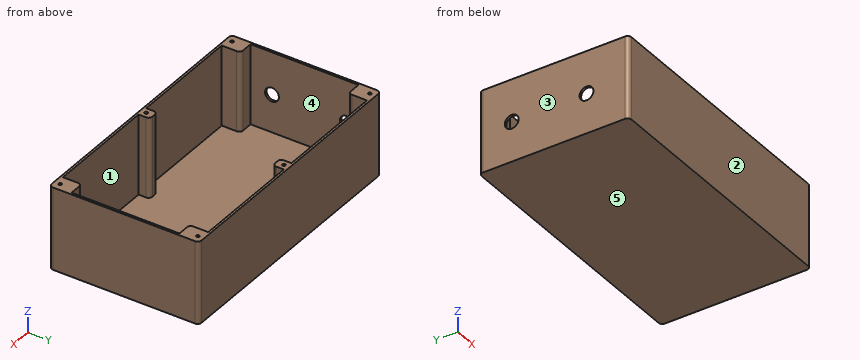
from build123d import *

# Parameters (mm, degrees)
F0_W     = 360
F0_H     = 200
F1_DEPTH = 110
F2_R     = 5
F3_T     = -3
F5_D     = 18.5
F5_DEPTH = 16.5
F5_TIP   = 5.557960726
F8_DEPTH = 107
F9_D     = 4.2
F9_DEPTH = 22.4
F9_TIP   = 1.2618073


with BuildPart() as f1:
    # F0 (on Top) → F1 (new body)
    with BuildSketch(Plane.XY):
        Rectangle(F0_W, F0_H)
    extrude(amount=F1_DEPTH)

    # F2
    f2_edges = [f1.edges().sort_by_distance(p)[0] for p in [
        (-180, 100, 55),
        (-180, -100, 55),
        (180, -100, 55),
        (180, 100, 55),
    ]]
    fillet(f2_edges, radius=F2_R)

    # F3
    f3_openings = [f1.faces().sort_by_distance(p)[0] for p in [
        (0, 0, 110),
    ]]
    offset(amount=F3_T, openings=f3_openings)

    # F5
    with Locations(Plane(origin=(-180, 0, 0), x_dir=(0, -1, 0), z_dir=(-1, 0, 0))):
        with Locations((-56.4456321299, 53.3652417362), (43.4474907815, 53.3652417362)):
            Hole(F5_D / 2, depth=F5_DEPTH)
            with Locations((0, 0, -(F5_DEPTH + F5_TIP / 2))):  # 118° drill point
                Cone(0, F5_D / 2, F5_TIP, mode=Mode.SUBTRACT)

    # F7 (on face) → F8 (join, through all)
    with BuildSketch(Plane.XY.offset(110)):
        with BuildLine():
            Line((-177, 95), (-177, 72))
            Line((-177, 72), (-162, 72))
            ThreePointArc((-162, 72), (-158.4644660941, 73.4644660941), (-157, 77))
            Line((-157, 77), (-157, 97))
            Line((-157, 97), (-175, 97))
            ThreePointArc((-175, 97), (-176.4142135624, 96.4142135624), (-177, 95))
        make_face()
        with BuildLine():
            Line((-175, -97), (-157, -97))
            Line((-157, -97), (-157, -77))
            ThreePointArc((-157, -77), (-158.4644660941, -73.4644660941), (-162, -72))
            Line((-162, -72), (-177, -72))
            Line((-177, -72), (-177, -95))
            ThreePointArc((-177, -95), (-176.4142135624, -96.4142135624), (-175, -97))
        make_face()
        with BuildLine():
            Line((7.5, 87), (7.5, 97))
            Line((7.5, 97), (-7.5, 97))
            Line((-7.5, 97), (-7.5, 87))
            ThreePointArc((-7.5, 87), (-6.0355339059, 83.4644660941), (-2.5, 82))
            Line((-2.5, 82), (2.5, 82))
            ThreePointArc((2.5, 82), (6.0355339059, 83.4644660941), (7.5, 87))
        make_face()
        with BuildLine():
            Line((-7.5, -97), (7.5, -97))
            Line((7.5, -97), (7.5, -87))
            ThreePointArc((7.5, -87), (6.0355339059, -83.4644660941), (2.5, -82))
            Line((2.5, -82), (-2.5, -82))
            ThreePointArc((-2.5, -82), (-6.0355339059, -83.4644660941), (-7.5, -87))
            Line((-7.5, -87), (-7.5, -97))
        make_face()
        with BuildLine():
            Line((157, -97), (175, -97))
            ThreePointArc((175, -97), (176.4142135624, -96.4142135624), (177, -95))
            Line((177, -95), (177, -72))
            Line((177, -72), (162, -72))
            ThreePointArc((162, -72), (158.4644660941, -73.4644660941), (157, -77))
            Line((157, -77), (157, -97))
        make_face()
        with BuildLine():
            Line((162, 72), (177, 72))
            Line((177, 72), (177, 95))
            ThreePointArc((177, 95), (176.4142135624, 96.4142135624), (175, 97))
            Line((175, 97), (157, 97))
            Line((157, 97), (157, 77))
            ThreePointArc((157, 77), (158.4644660941, 73.4644660941), (162, 72))
        make_face()
    extrude(amount=-F8_DEPTH)

    # F9
    with Locations(Plane.XY.offset(110)):
        with Locations((-170, -92), (-170, 92), (0, 92), (170, 92), (170, -92), (0, -92)):
            Hole(F9_D / 2, depth=F9_DEPTH)
            with Locations((0, 0, -(F9_DEPTH + F9_TIP / 2))):  # 118° drill point
                Cone(0, F9_D / 2, F9_TIP, mode=Mode.SUBTRACT)


solid = f1.part
Design review of the part built by this model. Coordinates are the model's own, in mm. Face numbers are marked on the shaded views. A direction names the side the tool comes from. Round coordinates to 2 decimals unless told otherwise and drop trailing zeros. Order: outer loops, then holes, each group sorted by start corner. A loop starts at its lowest first (then second) coordinate and runs counter-clockwise, first axis right, second up.
1) For L1, parallel to Y at x = -170, z = 95.75; L2, parallel to X at y = 87, z = 17; L3, parallel to X at y = -92, z = 101.25, list the stretches that pass through material, from the lowest coordinate up.
The answers:
L1: y = -100 to -94.1, -89.9 to -72, 72 to 89.9, 94.1 to 100
L2: x = -180 to -157, -7.5 to 7.5, 157 to 180
L3: x = -180 to -172.1, -167.9 to -157, -7.5 to -2.1, 2.1 to 7.5, 157 to 167.9, 172.1 to 180
2) Consider section A-A (x = 124). State the section outline as (y, z) points, plus the area to 3 significant figures.
The answers:
outline: (-100, 0) - (100, 0) - (100, 110) - (97, 110) - (97, 3) - (-97, 3) - (-97, 110) - (-100, 110) - close
area: 1,240 mm2
3) Draft analysis for pull direction X (two halves, no side actions). For the marked faces 1, 2 and 3, state which applies: released by +X, released by -X, zero draft, split by the parting line, or undercut.
The answers:
face 1: undercut
face 2: zero draft
face 3: released by -X
4) Clearance check with a flat-ended pin moving along its axis: pin 1 Ø15 at (y, z) = (-43.45, 53.37) entering from -X. State where the tip first meets the part, or that it passes through.
The answers:
pin 1: stops at x = 177
5) Consider section B-B (y = -22). State the section outline as (x, z) points.
The answers:
outline: (-180, 0) - (180, 0) - (180, 110) - (177, 110) - (177, 3) - (-177, 3) - (-177, 110) - (-180, 110) - close
6) Machinability: for the marked faces 4 and 5, which of the approach directions +Z, -Z, +X, -X, +Y, -Y give a long, thin tool a straight path to every point of the face, cutting with its end or side? Answer none if there is none.
The answers:
face 4: +Z
face 5: -Z, +X, -X, +Y, -Y
